from build123d import *

# Parameters (mm, degrees)
F0_W     = 57.347074
F0_H     = 21.480516
F1_DEPTH = 25.4
F3_DEPTH = 25.4
F5_DEPTH = 25.4


with BuildPart() as f1:
    # F0 (on Front) → F1 (new body)
    with BuildSketch(Plane.XZ):
        with Locations((28.673537, 23.155603)):
            Rectangle(F0_W, F0_H)
    extrude(amount=F1_DEPTH)

    # F2 (on Front) → F3 (cut)
    with BuildSketch(Plane.XZ):
        Polygon((57.347074, 33.895861), (0, 33.895861), (57.347074, 21.689083), align=None)
    extrude(amount=F3_DEPTH, mode=Mode.SUBTRACT)

    # F4 (on Front) → F5 (cut)
    with BuildSketch(Plane.XZ):
        Polygon((57.347074, 19.787414), (0, 12.415345), (57.347074, 12.415345), align=None)
    extrude(amount=F5_DEPTH, mode=Mode.SUBTRACT)


solid = f1.part
For this review, take the finished solid that the model builds, in its own axes (mm). Give positions to 0.01 mm unless a question says otherwise; leave off trailing zeros. Order: outer loops, then holes, each group sorted by start corner. A loop starts at its lowest first (then second) coordinate and runs counter-clockwise, first axis right, second up. Notation, with made-up numbers: M 66.5,57.5 L 95.5,57.5 A8 ccw 95.5,61.5 Z; hole C 35,82 d8. An arc over 180 degrees is marked long. Answer in a Markdown table with one row per item. Add a question column.
(1) For pin 1 (2 mm diameter, centred on x = 39.5, y = -12.5, fed in from +Z); pin 2 (2 mm diameter, centred on x = 10.5, y = -7.5, fed in from +Z); pin 3 (3 mm diameter, centred on x = 51.5, y = -11.5, fed in from -Z), all flat-tipped, find the tip position at first contact; note any pin that passes through.
(2) Consider section B-B on z = 19. State the section outline as (x, y) points.
(3) Consider section A-A on y = -21.75. State the section outline as (x, z) points.
(4) Wall thickness on probe 1 along Z at (x, y) = (26.5, -17); probe 2 along Z at (x, y) = (20, -1.5): over which ranges is each line inside the solid? List them lowest first. Write a range as [from, to].
Evaluation:
| question | item | result |
|---|---|---|
| 1 | pin 1 | stops at z = 25.7 |
| 1 | pin 2 | stops at z = 31.87 |
| 1 | pin 3 | stops at z = 18.84 |
| 2 | outline | M 0,-25.4 L 51.22,-25.4 L 51.22,0 L 0,0 Z |
| 3 | outline | M 0,12.42 L 57.35,19.79 L 57.35,21.69 L 0,33.9 Z |
| 4 | probe 1 | z = [15.82, 28.26] |
| 4 | probe 2 | z = [14.99, 29.64] |
